```python
from build123d import *

# Parameters (mm, degrees)
FILLET1_R                = 2
SKETCH5_R                = 8.5
SKETCH5_R_2              = 7
BOSS_EXTRUDE1_DEPTH      = 0.1
BOSS_EXTRUDE2_DEPTH      = 0.5
BOSS_EXTRUDE2_DEPTH_BACK = 0.5
SKETCH6_R                = 2
SKETCH6_R_2              = 1.5


with BuildPart() as part:
    # Sketch4 → Revolve1 (revolve)
    with BuildSketch(Plane(origin=(0, 0, 0), x_dir=(0, 0, -1), z_dir=(1, 0, 0))):
        Polygon((0, 0), (-3.75, 0), (-4.25, -0.5), (-4.75, 0), (-8.5, 0), (-8.5, -4), (0, -4), align=None)
    revolve(axis=Axis((0, 1.890471386, 0), (0, -1, 0)))

    # Fillet1
    fillet1_edges = [part.edges().sort_by_distance(p)[0] for p in [
        (0, 0, -8.5),
    ]]
    fillet(fillet1_edges, radius=FILLET1_R)



with BuildPart() as body_2:
    # Sketch5 → Boss-Extrude1 (new body)
    with BuildSketch(Plane.XZ.offset(4)):
        with Locations(Location((0, 0, 0), (0, 0, 90))):
            Circle(SKETCH5_R)
        with Locations(Location((0, 0, 0), (0, 0, 270))):
            Circle(SKETCH5_R_2, mode=Mode.SUBTRACT)
    extrude(amount=BOSS_EXTRUDE1_DEPTH)


with BuildPart() as part_1:
    add(part.part)

    add(body_2.part)  # Boss-Extrude2 merges body 2
    # Sketch6 → Boss-Extrude2 (add, two sides: drawn at the far end of the back side and taken through both)
    # profile 1 of 2: a face of its own
    with BuildSketch(Plane(origin=(0, 0, 0), x_dir=(0, 0, -1), z_dir=(1, 0, 0)).offset(-BOSS_EXTRUDE2_DEPTH_BACK)):
        with BuildLine():
            Line((18.982403574, 0), (0, 0))
            Line((0, 0), (0, -0.187703371))
            Line((0, -0.187703371), (7.006743711, -0.187703371))
            Line((7.006743711, -0.187703371), (8.5, -2))
            Line((8.5, -2), (16.888756121, -2.259364745))
            Line((16.888756121, -2.259364745), (20.011674859, -14.378186982))
            ThreePointArc((20.011674859, -14.378186982), (20.367556615, -12.653987247), (21.948404132, -11.879108109))
            Line((21.948404132, -11.879108109), (18.982403574, 0))
        make_face()
    # profile 2 of 2: a face of its own
    with BuildSketch(Plane(origin=(0, 0, 0), x_dir=(0, 0, -1), z_dir=(1, 0, 0)).offset(-BOSS_EXTRUDE2_DEPTH_BACK)):
        with Locations((21.948404132, -13.879108109)):
            Circle(SKETCH6_R)
        with Locations((21.948404132, -13.879108109)):
            Circle(SKETCH6_R_2, mode=Mode.SUBTRACT)
    extrude(amount=BOSS_EXTRUDE2_DEPTH + BOSS_EXTRUDE2_DEPTH_BACK)


solid = part_1.part
```
CAD build for the part. Positions are in the model's coordinates, mm. Give positions to 0.01 mm unless a question says otherwise; leave off trailing zeros. Order: outer loops, then holes, each group sorted by start corner. A loop starts at its lowest first (then second) coordinate and runs counter-clockwise, first axis right, second up. Notation, with made-up numbers: M 4.5,76 L 35.5,76 A20 ccw 35.5,82 Z; hole C 39.5,62 d6. An arc over 180 degrees is marked long. Put each result on its own line as item: value. Start each with the question number.
(1) Mould opens along Z. For faces 1 (the flat face through (0, -4, 0)), 2 (the flat face through (-0.007, -6.023, -20.486)), 3 (the flat face through (-7, -4.1, 2)) say: +Z half, -Z half, draft (parallel to the pull), parting line (faces both ways), or undercut.
(2) Saw through at A-A, the plane y = -3.5. Write the cut outline in (x, z).
(3) Saw through at B-B, the plane z = 0. Write the cut outline in (x, y).
(4) Drill centre lines: line 1 along X through (y, z) = (-4.05, 0); line 2 along X through (y, z) = (-2.25, -19.5); line 3 along Z through (x, y) = (-1, -1.25). Where is each one in solid material? Low to high.
(5) Saw through at C-C, the plane y = -13. Write the cut outline in (x, z).
(6) Saw through at D-D, the plane y = -9.75. Write the cut outline in (x, z).
(7) Flat gauge pins, fed straight in: pin 1 Ø5 at (y, z) = (-9, -9) entering from -X; pin 2 Ø1.5 at (y, z) = (-2.5, -13) entering from -X; pin 3 Ø5 at (y, z) = (-9.5, -18.5) entering from +X; pin 4 Ø8.5 at (x, z) = (3, 3) entering from -Y. Where does each tip first touch, or does it go through?
Check result:
1. face 1: undercut
1. face 2: -Z half
1. face 3: draft
2. outline: C 0,0 d17; M -0.5,-19.86 L 0.5,-19.86 L 0.5,-17.21 L -0.5,-17.21 Z
3. outline: M -8.5,-4.1 L -7,-4.1 L -7,-4 L 7,-4 L 7,-4.1 L 8.5,-4.1 L 8.5,-2 A2 ccw 6.5,0 L 4.75,0 L 4.25,-0.5 L 3.75,0 L -3.75,0 L -4.25,-0.5 L -4.75,0 L -6.5,0 A2 ccw -8.5,-2 Z
4. line 1: x = -8.5 to -7, 7 to 8.5
4. line 2: x = -0.5 to 0.5
4. line 3: z = -8.29 to 8.29
5. outline: M -0.5,-23.74 L 0.5,-23.74 L 0.5,-23.16 L -0.5,-23.16 Z; M -0.5,-20.73 L 0.5,-20.73 L 0.5,-19.66 L -0.5,-19.66 Z
6. outline: M -0.5,-21.42 L 0.5,-21.42 L 0.5,-18.82 L -0.5,-18.82 Z
7. pin 1: passes through
7. pin 2: stops at x = -0.5
7. pin 3: stops at x = 0.5
7. pin 4: stops at y = -4.1
